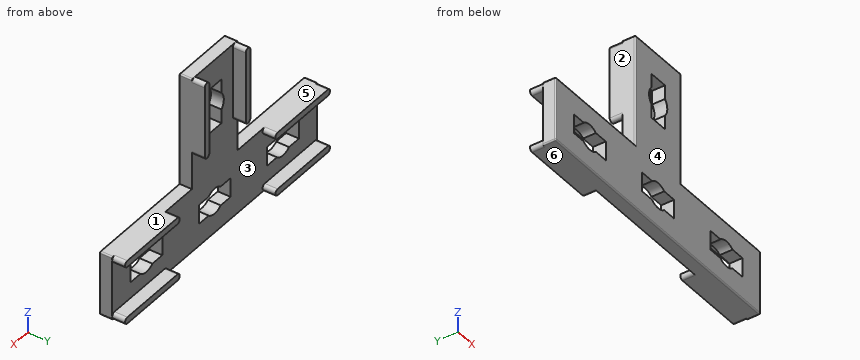
from build123d import *

# Parameters (mm, degrees)
EXTRUDE_1_DEPTH               = 2
EXTRUDE_2_DEPTH               = 2
PATTERN_LINEAR_1_COUNT        = 2
PATTERN_LINEAR_1_PITCH        = 33
PATTERN_LINEAR_1_COPY_1_DEPTH = 2
EXTRUDE_3_DEPTH               = 2
CUT_EXTRUDE_1_REACH           = 33.883
PATTERN_LINEAR_2_COUNT        = 2
PATTERN_LINEAR_2_PITCH        = 15
PATTERN_LINEAR_2_COL_COUNT    = 2
PATTERN_LINEAR_2_COL_PITCH    = 15
CUT_EXTRUDE_2_REACH           = 33.883
FILLET_1_R                    = 0.2


with BuildPart() as part:
    # 草图1 → 凸台-拉伸1 (new body)
    with BuildSketch(Plane(origin=(0, 0, 0), x_dir=(1, 0, 0), z_dir=(0, 1, 0))):
        Polygon((22.5, 5), (22.5, -5), (5, -5), (5, -22.5), (-5, -22.5), (-5, -5), (-22.5, -5), (-22.5, 5), align=None)
    extrude(amount=EXTRUDE_1_DEPTH)

    # 草图2 → 凸台-拉伸2 (add)
    with BuildSketch(Plane(origin=(0, 2, 0), x_dir=(1, 0, 0), z_dir=(0, 1, 0))):
        with BuildLine():
            Line((-22, 4), (-11, 4))
            ThreePointArc((-11, 4), (-10.5, 4.5), (-11, 5))
            Line((-11, 5), (-22, 5))
            ThreePointArc((-22, 5), (-22.5, 4.5), (-22, 4))
        make_face()
    extrude_2 = extrude(amount=EXTRUDE_2_DEPTH)

    # 镜向1: 凸台-拉伸2 across plane
    add(extrude_2.mirror(Plane.XY))

    # 阵列(线性)1: 凸台-拉伸2 ×2
    with Locations(*[(i * PATTERN_LINEAR_1_PITCH, 0, 0) for i in range(1, PATTERN_LINEAR_1_COUNT)]):
        add(extrude_2)

    # 阵列(线性)1 copy 1 sketch → 阵列(线性)1 copy 1 (add)
    with BuildSketch(Plane(origin=(33, 2, 0), x_dir=(1, 0, 0), z_dir=(0, 1, 0))):
        with BuildLine():
            Line((-22, -4), (-11, -4))
            ThreePointArc((-11, -4), (-10.5, -4.5), (-11, -5))
            Line((-11, -5), (-22, -5))
            ThreePointArc((-22, -5), (-22.5, -4.5), (-22, -4))
        make_face()
    extrude(amount=PATTERN_LINEAR_1_COPY_1_DEPTH)

    # 草图3 → 凸台-拉伸3 (add)
    with BuildSketch(Plane(origin=(0, 2, 0), x_dir=(1, 0, 0), z_dir=(0, 1, 0))):
        with BuildLine():
            Line((-4, -22), (-4, -11))
            ThreePointArc((-4, -11), (-4.5, -10.5), (-5, -11))
            Line((-5, -11), (-5, -22))
            ThreePointArc((-5, -22), (-4.5, -22.5), (-4, -22))
        make_face()
    extrude_3 = extrude(amount=EXTRUDE_3_DEPTH)

    # 镜向2: 凸台-拉伸3 across plane
    add(extrude_3.mirror(Plane(origin=(0, 0, 0), x_dir=(0, 0, 1), z_dir=(1, 0, 0))))

    # 草图4 → 切除-拉伸1 (cut, up to next)
    with BuildSketch(Plane(origin=(0, 2, 0), x_dir=(1, 0, 0), z_dir=(0, 1, 0)), mode=Mode.PRIVATE) as cut_extrude_1_sk1:
        with BuildLine():
            Line((3.5, 1.5), (3.5, -1.5))
            Line((3.5, -1.5), (1.322875656, -1.5))
            ThreePointArc((1.322875656, -1.5), (0, -2), (-1.322875656, -1.5))
            Line((-1.322875656, -1.5), (-3.5, -1.5))
            Line((-3.5, -1.5), (-3.5, 1.5))
            Line((-3.5, 1.5), (-1.322875656, 1.5))
            ThreePointArc((-1.322875656, 1.5), (0, 2), (1.322875656, 1.5))
            Line((1.322875656, 1.5), (3.5, 1.5))
        make_face()
    cut_extrude_1_tool1 = extrude(cut_extrude_1_sk1.sketch, amount=-CUT_EXTRUDE_1_REACH, mode=Mode.PRIVATE) & part.part
    cut_extrude_1 = cut_extrude_1_tool1.solids().sort_by_distance((0, 2, 0))[0]
    add(cut_extrude_1, mode=Mode.SUBTRACT)

    # 阵列(线性)2: 切除-拉伸1 ×2
    with Locations(*[(i * PATTERN_LINEAR_2_PITCH, 0, 0) for i in range(1, PATTERN_LINEAR_2_COUNT)]):
        add(cut_extrude_1, mode=Mode.SUBTRACT)

    # 阵列(线性)2 col: 切除-拉伸1 ×2
    with Locations(*[(-i * PATTERN_LINEAR_2_COL_PITCH, 0, 0) for i in range(1, PATTERN_LINEAR_2_COL_COUNT)]):
        add(cut_extrude_1, mode=Mode.SUBTRACT)

    # 草图5 → 切除-拉伸2 (cut, up to next)
    with BuildSketch(Plane(origin=(0, 2, 0), x_dir=(1, 0, 0), z_dir=(0, 1, 0)), mode=Mode.PRIVATE) as cut_extrude_2_sk1:
        with BuildLine():
            Line((1.5, -11.5), (-1.5, -11.5))
            Line((-1.5, -11.5), (-1.5, -13.677124344))
            ThreePointArc((-1.5, -13.677124344), (-2, -15), (-1.5, -16.322875656))
            Line((-1.5, -16.322875656), (-1.5, -18.5))
            Line((-1.5, -18.5), (1.5, -18.5))
            Line((1.5, -18.5), (1.5, -16.322875656))
            ThreePointArc((1.5, -16.322875656), (2, -15), (1.5, -13.677124344))
            Line((1.5, -13.677124344), (1.5, -11.5))
        make_face()
    cut_extrude_2_tool1 = extrude(cut_extrude_2_sk1.sketch, amount=-CUT_EXTRUDE_2_REACH, mode=Mode.PRIVATE) & part.part
    add(cut_extrude_2_tool1.solids().sort_by_distance((0, 2, 15))[0], mode=Mode.SUBTRACT)

    # 圆角1
    fillet_1_edges = [part.edges().sort_by_distance(p)[0] for p in [
        (22.5, 1, 5),
        (22.5, 1, -5),
        (-22.5, 1, -5),
        (-22.5, 1, 5),
        (5, 1, 22.5),
        (-5, 1, 22.5),
        (-22.5, 0, 0),
        (22.5, 0, 0),
        (0, 0, 22.5),
        (5, 0, 13.75),
        (-5, 0, 13.75),
        (-13.75, 0, 5),
        (13.75, 0, 5),
        (0, 0, -5),
    ]]
    fillet(fillet_1_edges, radius=FILLET_1_R)


solid = part.part
Can you work these out from the model? Positions are in its coordinate system, mm. Face numbers are marked on the shaded views. A direction names the side the tool comes from. Round coordinates to 2 decimals unless told otherwise and drop trailing zeros. Write each loop counter-clockwise with the first axis right and the second up, starting at its lowest first coordinate (ties: lowest second). Pieces come first, ordered by that corner, then holes. Notation, with made-up numbers: (89, -31.75) - (129, -31.75) arc R29 ccw to (129, 1.25) - close; hole circle Ø7 at (-38.5, 0). An arc over 180 degrees is marked (long way). Write each question's results on one line, items separated by ' | '. Start each with the question number.
1) Suppose I cut it at A-A (z = 19.75). List the corners of the cut face in (x, y) for me, and give its area (3 significant figures).
2) We'd pull the mould along Z, two halves only. Please class the marked faces 3, 4, 5 and 6: released by +Z, released by -Z, zero draft, split by the parting line, or undercut.
3) For pin 1 Ø2 at (y, z) = (1.5, 10) entering from -X; pin 2 Ø1.6 at (y, z) = (3, 17) entering from +X; pin 3 Ø1 at (x, y) = (-17, 1.5) entering from +Z; pin 4 Ø12 at (x, z) = (-11.5, 2) entering from +Y, each with a flat end and sliding along its axis, tell me the tip position at first contact or that it passes through.
4) Please list where these lines run through material, in increasing order: line 1 (X direction, y = 2.85, z = 20); line 2 (Z direction, x = -17.5, y = 1).
5) Which directions (+Z, -Z, +X, -X, +Y, -Y) give clear straight access to the entire face, cutting with the end or side of a thin tool? Please do the marked faces 1 and 2.
6) Suppose I cut it at C-C (y = 0.95). Give the number of separate pieces and of enclosed holes in the cut face, and give its area (3 significant figures).
7) Suppose I cut it at B-B (x = 10). List the corners of the cut face in (y, z) for me.
Here are the results:
1) outline: (-5, 0.2) arc R0.2 ccw to (-4.8, 0) - (4.8, 0) arc R0.2 ccw to (5, 0.2) - (5, 4) - (4, 4) - (4, 2) - (-4, 2) - (-4, 4) - (-5, 4) - close | area: 24.0 mm2
2) face 3: undercut | face 4: zero draft | face 5: released by +Z | face 6: released by -Z
3) pin 1: stops at x = -5 | pin 2: stops at x = 5 | pin 3: stops at z = 5 | pin 4: stops at y = 4
4) line 1: x = -5 to -4, 4 to 5 | line 2: z = -5 to -1.5, 1.5 to 5
5) face 1: +Z, +X, +Y, -Y | face 2: +Z, -X, +Y, -Y
6) separate pieces: 1 | enclosed holes: 4 | area: 534 mm2
7) outline: (0, -4.8) arc R0.2 ccw to (0.2, -5) - (2, -5) - (2, 5) - (0.2, 5) arc R0.2 ccw to (0, 4.8) - close
